For this review, take the finished solid that the model builds, in its own axes (mm). A direction names the side the tool comes from. Coordinates: 2 decimals unless noted, no trailing zeros. Loops run counter-clockwise (first coordinate to the right, second up) from the corner with the lowest first, then second, coordinate; pieces in that order, holes last. Notation, with made-up numbers: (87.25, 82) - (96.25, 82) arc R10 cw to (96.25, 98) - close; hole circle Ø11 at (33, 61.25). An arc over 180 degrees is marked (long way). Answer as a JSON object with one key per item and string values. Group by question number.
Item 1: Clearance check with flat-ended pins moving along their axes: pin 1 (3 mm diameter, centred on x = 15.5, z = -11, fed in from +Y); pin 2 (6 mm diameter, centred on x = 14, y = 9, fed in from +Z); pin 3 (12 mm diameter, centred on x = 28.5, z = -4.5, fed in from +Y). State where each tip first meets the part, or that it passes through.
Item 2: Mouldability with a two-part tool opening along X and no side actions: class faces 1 (the cylindrical face through (-33.5, 3.2, -0.1)), 2 (the cylindrical face through (18.5, 9.7, 0.1)), 3 (the cylindrical face through (-23.794, 3.204, -1.407)) as released by +X, released by -X, zero draft, split by the parting line, or undercut.
Item 3: We need section A-A (x = 0). Give the boundary of the cut face in (y, z).
Item 4: We need section C-C (y = 10.75). Give the boundary of the cut face in (x, z), then the cut area to 3 significant figures.
Item 5: Tool access review of faces 4 (the cylindrical face through (-18.5, 9.7, -0.1)), 5 (the flat face through (-9.3, 13, 4.4)), 6 (the flat face through (24.452, 3.204, 7.237)): name each direction out of +Z, -Z, +X, -X, +Y, -Y from which nothing blocks a thin tool from reaching the whole face with its end or side.
Item 6: To check wall thickness, follow line 1 (Y direction, x = 11.5, z = -14); line 2 (Z direction, x = 26.5, y = 4.5); line 3 (Y direction, x = -28, z = 3.5). State the ranges of each line that lie inside material, in increasing order.
Item 7: We need section D-D (x = 26.5). Give the boundary of the cut face in (y, z).
Item 8: We need section B-B (z = 0). Give the boundary of the cut face in (x, y), then the cut area to 3 significant figures.
from build123d import *

# Parameters (mm, degrees)
SKETCH3_R           = 3.05
BOSS_EXTRUDE1_DEPTH = 6.5
BOSS_EXTRUDE2_DEPTH = 6.5
SKETCH5_R           = 10
BOSS_EXTRUDE3_DEPTH = 5.6
SKETCH6_R           = 7.5
CUT_EXTRUDE1_DEPTH  = 44.694507664


with BuildPart() as part:
    # Sketch3 → Boss-Extrude1 (new body)
    # profile 1 of 5: a face of its own
    with BuildSketch(Plane(origin=(0, 0, 0), x_dir=(1, 0, 0), z_dir=(0, 1, 0))):
        with BuildLine():
            Line((0, -17.966933692), (-18.56176162, -9.821456387))
            ThreePointArc((-18.56176162, -9.821456387), (0, -21), (18.56176162, -9.821456387))
            Line((18.56176162, -9.821456387), (0, -17.966933692))
        make_face()
    # profile 2 of 5: a face of its own
    with BuildSketch(Plane(origin=(0, 0, 0), x_dir=(1, 0, 0), z_dir=(0, 1, 0))):
        with BuildLine():
            Line((0, 17.966933692), (-18.56176162, 9.821456387))
            ThreePointArc((-18.56176162, 9.821456387), (-21, 0), (-18.56176162, -9.821456387))
            Line((-18.56176162, -9.821456387), (0, -17.966933692))
            Line((0, -17.966933692), (18.56176162, -9.821456387))
            ThreePointArc((18.56176162, -9.821456387), (20.381327165, -5.059792782), (21, 0))
            ThreePointArc((21, 0), (20.381327165, 5.059792782), (18.56176162, 9.821456387))
            Line((18.56176162, 9.821456387), (0, 17.966933692))
        make_face()
    # profile 3 of 5: a face of its own
    with BuildSketch(Plane(origin=(0, 0, 0), x_dir=(1, 0, 0), z_dir=(0, 1, 0))):
        with BuildLine():
            ThreePointArc((18.56176162, 9.821456387), (0, 21), (-18.56176162, 9.821456387))
            Line((-18.56176162, 9.821456387), (0, 17.966933692))
            Line((0, 17.966933692), (18.56176162, 9.821456387))
        make_face()
    # profile 4 of 5: a face of its own
    with BuildSketch(Plane(origin=(0, 0, 0), x_dir=(1, 0, 0), z_dir=(0, 1, 0))):
        with BuildLine():
            Line((30.509208106, 4.578545925), (18.56176162, 9.821456387))
            ThreePointArc((18.56176162, 9.821456387), (20.381327165, 5.059792782), (21, 0))
            ThreePointArc((21, 0), (20.381327165, -5.059792782), (18.56176162, -9.821456387))
            Line((18.56176162, -9.821456387), (30.509208106, -4.578545925))
            ThreePointArc((30.509208106, -4.578545925), (33.5, 0), (30.509208106, 4.578545925))
        make_face()
        with Locations(Location((26.5, 0, 0), (0, 0, 90))):
            Circle(SKETCH3_R, mode=Mode.SUBTRACT)
    # profile 5 of 5: a face of its own
    with BuildSketch(Plane(origin=(0, 0, 0), x_dir=(1, 0, 0), z_dir=(0, 1, 0))):
        with BuildLine():
            Line((-18.56176162, 9.821456387), (-30.509208106, 4.578545925))
            ThreePointArc((-30.509208106, 4.578545925), (-33.5, 0), (-30.509208106, -4.578545925))
            Line((-30.509208106, -4.578545925), (-18.56176162, -9.821456387))
            ThreePointArc((-18.56176162, -9.821456387), (-21, 0), (-18.56176162, 9.821456387))
        make_face()
        with Locations(Location((-26.5, 0, 0), (0, 0, 90))):
            Circle(SKETCH3_R, mode=Mode.SUBTRACT)
    extrude(amount=BOSS_EXTRUDE1_DEPTH)

    # Sketch4 → Boss-Extrude2 (add)
    with BuildSketch(Plane(origin=(0, 6.5, 0), x_dir=(1, 0, 0), z_dir=(0, 1, 0))):
        with BuildLine():
            ThreePointArc((20.363207547, 5.132229378), (0, 21), (-20.363207547, 5.132229378))
            ThreePointArc((-20.363207547, 5.132229378), (-18.5, 0), (-20.363207547, -5.132229378))
            ThreePointArc((-20.363207547, -5.132229378), (0, -21), (20.363207547, -5.132229378))
            ThreePointArc((20.363207547, -5.132229378), (18.5, 0), (20.363207547, 5.132229378))
        make_face()
    extrude(amount=BOSS_EXTRUDE2_DEPTH)

    # Sketch5 → Boss-Extrude3 (add)
    with BuildSketch(Plane(origin=(0, 13, 0), x_dir=(1, 0, 0), z_dir=(0, 1, 0))):
        with Locations(Location((0, 0, 0), (0, 0, 270))):
            Circle(SKETCH5_R)
    extrude(amount=BOSS_EXTRUDE3_DEPTH)

    # Sketch6 → Cut-Extrude1 (cut, through all)
    with BuildSketch(Plane(origin=(0, 18.6, 0), x_dir=(1, 0, 0), z_dir=(0, 1, 0))):
        with Locations(Location((0, 0, 0), (0, 0, 270))):
            Circle(SKETCH6_R)
    extrude(amount=-CUT_EXTRUDE1_DEPTH, mode=Mode.SUBTRACT)


solid = part.part
Check sheet entries:
{
 "1": {"pin 1": "stops at y = 13", "pin 2": "stops at z = 17.89", "pin 3": "stops at y = 6.5"},
 "2": {"face 1": "released by -X", "face 2": "released by +X", "face 3": "undercut"},
 "3": {"outline": "(0, -21) - (13, -21) - (13, -10) - (18.6, -10) - (18.6, -7.5) - (0, -7.5) - close; (0, 7.5) - (18.6, 7.5) - (18.6, 10) - (13, 10) - (13, 21) - (0, 21) - close"},
 "4": {"outline": "(-20.36, -5.13) arc R21 ccw to (20.36, -5.13) arc R8 cw to (20.36, 5.13) arc R21 ccw to (-20.36, 5.13) arc R8 cw to start; hole circle Ø15 at (0, 0)", "area": "1,170 mm2"},
 "5": {"face 4": "-X, +Y", "face 5": "+Y", "face 6": "+Z, +X, +Y, -Y"},
 "6": {"line 1": "y = 0 to 13", "line 2": "z = -6.34 to -3.05, 3.05 to 6.34", "line 3": "y = 0 to 6.5"},
 "7": {"outline": "(0, -6.34) - (6.5, -6.34) - (6.5, -3.05) - (0, -3.05) - close; (0, 3.05) - (6.5, 3.05) - (6.5, 6.34) - (0, 6.34) - close"},
 "8": {"outline": "(-33.5, 0) - (-29.55, 0) - (-29.55, 6.5) - (-33.5, 6.5) - close; (-23.45, 0) - (-7.5, 0) - (-7.5, 18.6) - (-10, 18.6) - (-10, 13) - (-18.5, 13) - (-18.5, 6.5) - (-23.45, 6.5) - close; (7.5, 0) - (23.45, 0) - (23.45, 6.5) - (18.5, 6.5) - (18.5, 13) - (10, 13) - (10, 18.6) - (7.5, 18.6) - close; (29.55, 0) - (33.5, 0) - (33.5, 6.5) - (29.55, 6.5) - close", "area": "430 mm2"}
}
